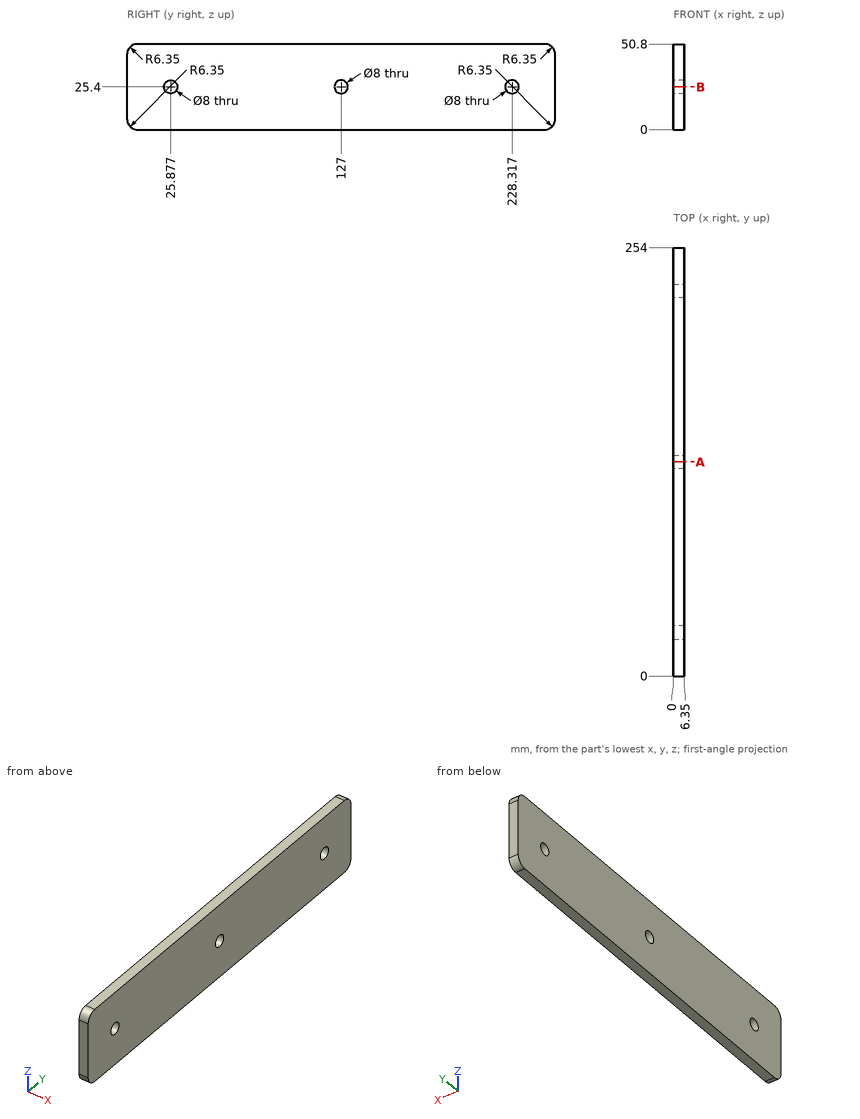
Geometry: see drawing. Coordinates: mm, zero at the bounding-box minimum. Give positions to 0.01 mm unless a question says otherwise; leave off trailing zeros. Write each loop counter-clockwise with the first axis right and the second up, starting at its lowest first coordinate (ties: lowest second). Pieces come first, ordered by that corner, then holes. Notation, with made-up numbers: (89, -6.75) - (108, -6.75) arc R6 ccw to (108, -1.75) - close; hole circle Ø10 at (-9, 65). An arc over 180 degrees is marked (long way). Return JSON: item names as keys, results as strings. Group by question number.
1) Section A-A on y = 127. Return the cut outline in (x, z), plus the area to 3 significant figures.
2) Line query: line 1 (Z direction, x = 2.75, y = 127); line 2 (Z direction, x = 1.25, y = 232); line 3 (Y direction, x = 1.25, z = 3.5) (1 decimal). Output: solid intervals per line, ascending.
3) Section B-B on z = 25.4. Return the cut outline in (x, y), plus the area to 3 significant figures.
Filled in:
{
 "1": {"outline": "(0, 0) - (6.35, 0) - (6.35, 21.4) - (0, 21.4) - close; (0, 29.4) - (6.35, 29.4) - (6.35, 50.8) - (0, 50.8) - close", "area": "272 mm^2"},
 "2": {"line 1": "z = 0 to 21.4, 29.4 to 50.8", "line 2": "z = 0 to 23.84, 26.96 to 50.8", "line 3": "y = 0.7 to 253.3"},
 "3": {"outline": "(0, 0) - (6.35, 0) - (6.35, 21.88) - (0, 21.88) - close; (0, 29.88) - (6.35, 29.88) - (6.35, 123) - (0, 123) - close; (0, 131) - (6.35, 131) - (6.35, 224.32) - (0, 224.32) - close; (0, 232.32) - (6.35, 232.32) - (6.35, 254) - (0, 254) - close", "area": "1,460 mm^2"}
}
